Geometry: final body of the model. Coordinates: model frame, mm. Face numbers are marked on the shaded views. A direction names the side the tool comes from. Give positions to 0.01 mm unless a question says otherwise; leave off trailing zeros. Write each loop counter-clockwise with the first axis right and the second up, starting at its lowest first coordinate (ties: lowest second). Pieces come first, ordered by that corner, then holes.
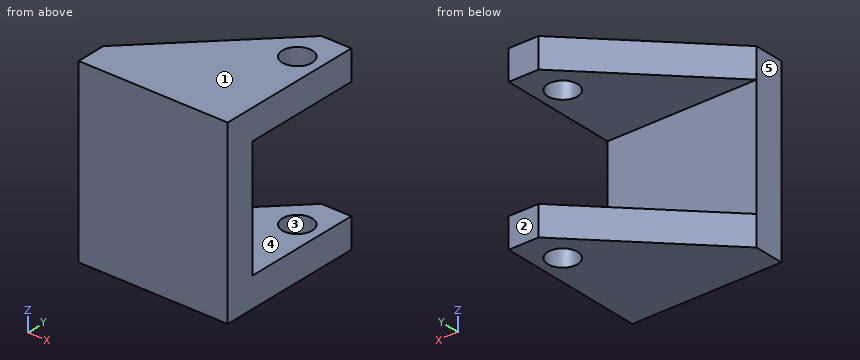
from build123d import *

# Parameters (mm, degrees)
BOSS_EXTRUDE1_DEPTH = 38.1
SKETCH2_W           = 25.4
SKETCH2_H           = 25.4
CUT_EXTRUDE1_DEPTH  = 38.1
SKETCH3_R           = 3.175
CUT_EXTRUDE2_DEPTH  = 38.1


with BuildPart() as part:
    # Sketch1 → Boss-Extrude1 (new body)
    with BuildSketch(Plane.XY):
        Polygon((-31.75, 0), (0, 0), (0, 31.75), (-6.35, 31.75), (-31.75, 6.35), align=None)
    extrude(amount=BOSS_EXTRUDE1_DEPTH)

    # Sketch2 → Cut-Extrude1 (cut)
    with BuildSketch(Plane(origin=(0, 0, 0), x_dir=(0, 0, -1), z_dir=(1, 0, 0))):
        with Locations((-19.05, 19.05)):
            Rectangle(SKETCH2_W, SKETCH2_H)
    extrude(amount=-CUT_EXTRUDE1_DEPTH, mode=Mode.SUBTRACT)

    # Sketch3 → Cut-Extrude2 (cut)
    with BuildSketch(Plane.XY.offset(38.1)):
        with Locations((-5.08, 24)):
            Circle(SKETCH3_R)
    extrude(amount=-CUT_EXTRUDE2_DEPTH, mode=Mode.SUBTRACT)


solid = part.part
Q1. Pin query (flat end, axial travel): P1, Ø6, axis at y = 11, z = 14, coming from the +X side; P2, Ø12.5, axis at x = -16, z = 14.5, coming from the +Y side. Return the tip coordinate at first contact, or that it passes through.
Filled sheet:
P1: passes through
P2: stops at y = 6.35
Q2. Section D-D on x = -5.08. Output: boundary loops of the cut face in (y, z) (3 decimals), plus the area to 3 significant figures.
Filled sheet:
outline: (0, 0) - (20.825, 0) - (20.825, 6.35) - (6.35, 6.35) - (6.35, 31.75) - (20.825, 31.75) - (20.825, 38.1) - (0, 38.1) - close; (27.175, 0) - (31.75, 0) - (31.75, 6.35) - (27.175, 6.35) - close; (27.175, 31.75) - (31.75, 31.75) - (31.75, 38.1) - (27.175, 38.1) - close
area: 484 mm2
Q3. Section A-A on y = 16. Output: boundary loops of the cut face in (x, z).
Filled sheet:
outline: (-22.1, 0) - (0, 0) - (0, 6.35) - (-22.1, 6.35) - close; (-22.1, 31.75) - (0, 31.75) - (0, 38.1) - (-22.1, 38.1) - close
Q4. Section B-B on x = -28. Output: boundary loops of the cut face in (y, z).
Filled sheet:
outline: (0, 0) - (10.1, 0) - (10.1, 6.35) - (6.35, 6.35) - (6.35, 31.75) - (10.1, 31.75) - (10.1, 38.1) - (0, 38.1) - close
Q5. Section C-C on y = 24. Output: boundary loops of the cut face in (x, z) (3 decimals).
Filled sheet:
outline: (-14.1, 0) - (-8.255, 0) - (-8.255, 6.35) - (-14.1, 6.35) - close; (-14.1, 31.75) - (-8.255, 31.75) - (-8.255, 38.1) - (-14.1, 38.1) - close; (-1.905, 0) - (0, 0) - (0, 6.35) - (-1.905, 6.35) - close; (-1.905, 31.75) - (0, 31.75) - (0, 38.1) - (-1.905, 38.1) - close
Q6. Ray query, line 1 along Y through (x, z) = (-5.08, 36.5) (3 decimals); line 2 along Z through (x, y) = (-4, 16); line 3 along Y through (x, z) = (-6, 7.5). Return the intervals inside material, ascending.
Filled sheet:
line 1: y = 0 to 20.825, 27.175 to 31.75
line 2: z = 0 to 6.35, 31.75 to 38.1
line 3: y = 0 to 6.35
Q7. Pull-direction query (Y, two-part tool) for the marked faces 1, 2 and 3; classes: released by +Y, released by -Y, zero draft, split by the parting line, or undercut.
Filled sheet:
face 1: zero draft
face 2: released by +Y
face 3: undercut
Q8. Access query for the marked faces 4 and 5. Directions: +Z, -Z, +X, -X, +Y, -Y. A direction counts if a zero-diameter tool reaches every point of the face in a straight line with its end or side. Return the directions, or none.
Filled sheet:
face 4: +X, -X, +Y
face 5: +Z, -Z, -X, +Y, -Y
